Geometry: final body of the model. Coordinates: model frame, mm. A direction names the side the tool comes from. Give positions to 0.01 mm unless a question says otherwise; leave off trailing zeros. Write each loop counter-clockwise with the first axis right and the second up, starting at its lowest first coordinate (ties: lowest second). Pieces come first, ordered by that corner, then holes.
Q1. Section C-C (z = 2.5). Return the cut outline in (x, y), plus the area to 3 significant figures.
Q2. Mould query, pull axis X, two halves, no side actions, for faces 1 (the cylindrical face through (-0.9, 2.86, 6.33)), 2 (the cylindrical face through (0.66, -14.985, 11.979)), 3 (the flat face through (3, 3, 0)). Classes: +X half, -X half, draft (parallel to the pull), parting line (faces both ways), or undercut.
Q3. Section A-A (z = 11). Return the cut outline in (x, y), plus the area to 3 significant figures.
Q4. Line query: line 1 (Y direction, x = 0, z = 5.5); line 2 (X direction, y = -3, z = 3). Output: solid intervals per line, ascending.
Q5. Reachability of faces 4 (the cylindrical face through (-2.681, 6.466, 3.212)), 5 (the cylindrical face through (-0.369, -4.898, 3.673)) from +Z, -Z, +X, -X, +Y, -Y: full face, straight path, thin tool, end or side. Return the list, or none.
Q6. Pin query (flat end, axial travel): pin 1 Ø1.5 at (x, y) = (12, 10) entering from +Z; pin 2 Ø3 at (x, z) = (0, 2.5) entering from +Y; pin 3 Ø4 at (y, z) = (-2.5, 6) entering from +X; pin 4 Ø2 at (y, z) = (9.5, 7) entering from -X. Return the tip coordinate at first contact, or that it passes through.
Q7. Section B-B (z = 4.5). Return the cut outline in (x, y), plus the area to 3 significant figures.
Autodesk Inventor part; units mm, degrees
ref_plane "YZ Plane" through (0, 0, 0) normal (1, 0, 0) x (0, 1, 0)
ref_plane "XZ Plane" through (0, 0, 0) normal (0, 1, 0) x (-1, 0, 0)
ref_plane "XY Plane" through (0, 0, 0) normal (0, 0, 1) x (1, 0, 0)
sketch "Skizze1" plane through (0, 0, 0) normal (1, 0, 0) x (0, 1, 0)
  line L0 (0, 0) -> (0, 67.4576) construction
  line L1 (3, 0) -> (3, 12)
  line L2 (3, 12) -> (0, 12)
  line L3 (0, 12) -> (0, 15)
  line L4 (15, 14) -> (15, 10)
  line L5 (7, 6) -> (7, 0)
  line L6 (7, 0) -> (3, 0)
  arc A0 (15, 10) -> (7, 6) centre (15, 0) ccw
  line L7 (15, 10) -> (23.1737, 10) construction
  arc A1 (15, 14) -> (0, 15) centre (0, -98) ccw
  line L8 (0, 15) -> (-13.142, 15) construction
  dimension "d0" = 6
  dimension "d1" = 14
  dimension "d2" = 30
  dimension "d3" = 6
  dimension "d5" = 4
  dimension "d6" = 12
  dimension "d12" = 10
  dimension "d13" = 15
revolve "Umdrehung1" add sketch "Skizze1" angle 360 about axis through (0, 0, 0) along (0, 0, 1)
chamfer "Fase1" distance 0.5 angle 45 4 edges at (0, -7, 0) (0, -3, 0) (0, -15, 10) (0, -15, 14)
sketch "Skizze2" plane through (0, 0, 0) normal (0, 1, 0) x (-1, 0, 0)
  line L0 (6.5, 0) -> (-6.5, 0)
  point P0 (0, 0)
  point P1 (0, 2.5)
  point P2 (0, 0)
  dimension "d14" = 2.5
hole "Bohrung1" at (0, 0, 2.5) direction (0, -1, 0) diameter 2.459 end through all
properties part number "EW_Drehknopf" material "Messing, weicher Gelbton"
Computed:
1. outline: (-1.23, -6.89) - (-1.23, -2.74) arc R3 cw (long way) to (1.23, -2.74) - (1.23, -6.89) arc R7 ccw (long way) to start
1. area: 116 mm2
2. face 1: undercut
2. face 2: parting line
2. face 3: draft
3. outline: circle Ø30 at (0, 0); hole circle Ø6 at (0, 0)
3. area: 679 mm2
4. line 1: y = -7 to -3, 3 to 7
4. line 2: x = -6.32 to -1.12, 1.12 to 6.32
5. face 4: -Z
5. face 5: -Y
6. pin 1: stops at z = 13.65
6. pin 2: stops at y = 7
6. pin 3: stops at x = 8.7
6. pin 4: passes through
7. outline: circle Ø14 at (0, 0); hole circle Ø6 at (0, 0)
7. area: 126 mm2
